from build123d import *

# Parameters (mm, degrees)
SKETCH1_W           = 18
SKETCH1_H           = 80
BOSS_EXTRUDE1_DEPTH = 5
SKETCH2_W           = 5
SKETCH2_H           = 25
BOSS_EXTRUDE2_DEPTH = 5
SKETCH3_W           = 9
SKETCH3_H           = 5
BOSS_EXTRUDE3_DEPTH = 5
SKETCH4_W           = 10
SKETCH4_H           = 5
BOSS_EXTRUDE4_DEPTH = 5
SKETCH5_R           = 2.1
CUT_EXTRUDE1_DEPTH  = 5
BOSS_EXTRUDE5_DEPTH = 5
SKETCH7_W           = 5
SKETCH7_H           = 4.2
CUT_EXTRUDE2_DEPTH  = 5


with BuildPart() as part:
    # Sketch1 → Boss-Extrude1 (new body)
    with BuildSketch(Plane.XY):
        with Locations((-9, 40)):
            Rectangle(SKETCH1_W, SKETCH1_H)
    extrude(amount=BOSS_EXTRUDE1_DEPTH)

    # Sketch2 → Boss-Extrude2 (add)
    with BuildSketch(Plane(origin=(0, 0, 0), x_dir=(-1, 0, 0), z_dir=(0, 0, -1))):
        with Locations((-2.5, 62.5)):
            Rectangle(SKETCH2_W, SKETCH2_H)
        with Locations((-2.5, 17.5)):
            Rectangle(SKETCH2_W, SKETCH2_H)
        with Locations((20.5, 17.5)):
            Rectangle(SKETCH2_W, SKETCH2_H)
        with Locations((20.5, 62.5)):
            Rectangle(SKETCH2_W, SKETCH2_H)
    extrude(amount=-BOSS_EXTRUDE2_DEPTH)

    # Sketch3 → Boss-Extrude3 (add)
    with BuildSketch(Plane.XZ):
        with Locations((-4.5, 2.5)):
            Rectangle(SKETCH3_W, SKETCH3_H)
    extrude(amount=BOSS_EXTRUDE3_DEPTH)

    # Sketch4 → Boss-Extrude4 (add)
    with BuildSketch(Plane(origin=(0, 0, 0), x_dir=(-1, 0, 0), z_dir=(0, 0, -1))):
        with Locations((5, 82.5)):
            Rectangle(SKETCH4_W, SKETCH4_H)
    extrude(amount=-BOSS_EXTRUDE4_DEPTH)

    # Sketch5 → Cut-Extrude1 (cut)
    with BuildSketch(Plane(origin=(0, 0, 0), x_dir=(-1, 0, 0), z_dir=(0, 0, -1))):
        with Locations((-2.5, 62.5)):
            Circle(SKETCH5_R)
        with Locations((-2.5, 17.5)):
            Circle(SKETCH5_R)
    extrude(amount=-CUT_EXTRUDE1_DEPTH, mode=Mode.SUBTRACT)

    # Sketch6 → Boss-Extrude5 (add)
    with BuildSketch(Plane(origin=(0, 0, 0), x_dir=(-1, 0, 0), z_dir=(0, 0, -1))):
        with BuildLine():
            Line((-5, 66.830127019), (-5, 58.169872981))
            ThreePointArc((-5, 58.169872981), (-7.5, 62.5), (-5, 66.830127019))
        make_face()
        with BuildLine():
            Line((-5, 13.169872981), (-5, 21.830127019))
            ThreePointArc((-5, 21.830127019), (-7.5, 17.5), (-5, 13.169872981))
        make_face()
    extrude(amount=-BOSS_EXTRUDE5_DEPTH)

    # Sketch7 → Cut-Extrude2 (cut)
    with BuildSketch(Plane.XY.offset(5)):
        Polygon((-13, 45), (-13, 42.1), (-13, 37.9), (-13, 35), (-3, 35), (-3, 45), align=None)
        with Locations((-15.5, 40)):
            Rectangle(SKETCH7_W, SKETCH7_H)
    extrude(amount=-CUT_EXTRUDE2_DEPTH, mode=Mode.SUBTRACT)


solid = part.part
The listing builds one solid part. Answer for the finished solid, in the listing's coordinates (mm). A direction names the side the tool comes from. Coordinates: 2 decimals unless noted, no trailing zeros. Order: outer loops, then holes, each group sorted by start corner. A loop starts at its lowest first (then second) coordinate and runs counter-clockwise, first axis right, second up. Notation, with made-up numbers: M 47.5,-22.5 L 70.5,-22.5 A28 ccw 70.5,9.5 Z; hole C -2.5,61.5 d1. An arc over 180 degrees is marked long. Use CSV: the item, a comma, the result in double quotes.
Q1. Determine the mould class of faces 5 (the flat face through (-20, 30, 2)), 6 (the flat face through (-23, 62, 2)), 7 (the cylindrical face through (1.37, 19.27, 2.46)) for opening direction X: pulls with the +X half, pulls with the -X half, needs draft (parallel to the pull), parting line crosses it, or undercut.
Here are the results:
face 5,"needs draft"
face 6,"pulls with the -X half"
face 7,"undercut"
Q2. Section C-C (y = 62.5) is taken. Determine the outline of the cut face in (x, z), then the cut area to 4 significant figures.
Here are the results:
outline,"M -23,0 L 0.4,0 L 0.4,5 L -23,5 Z; M 4.6,0 L 7.5,0 L 7.5,5 L 4.6,5 Z"
area,"131.5 mm2"
Q3. Section B-B (x = 2.5) is taken. Determine the outline of the cut face in (y, z).
Here are the results:
outline,"M 5,0 L 15.4,0 L 15.4,5 L 5,5 Z; M 19.6,0 L 30,0 L 30,5 L 19.6,5 Z; M 50,0 L 60.4,0 L 60.4,5 L 50,5 Z; M 64.6,0 L 75,0 L 75,5 L 64.6,5 Z"
Q4. Straight lines are drawn through the part: L1, parallel to Y at x = 2.5, z = 1; L2, parallel to Y at x = -19.5, z = 3.4; L3, parallel to Y at x = -11.5, z = 0.3. For each, find the intervals that lie inside material, in ascending order.
Here are the results:
L1,"5 to 15.4, 19.6 to 30, 50 to 60.4, 64.6 to 75"
L2,"5 to 30, 50 to 75"
L3,"0 to 35, 45 to 80"
Q5. A tool of negligible diameter and unlimited length cuts with its end or side. For faces 1 (the flat face through (-14, 0, 2)), 2 (the flat face through (-16, 37.9, 3)), 3 (the flat face through (-13, 36, 3)), 4 (the flat face through (0, 0, 2)), from which of +Z, -Z, +X, -X, +Y, -Y can it reach the whole face along a straight path? Write none if from no direction.
Here are the results:
face 1,"+Z, -Z, -X, -Y"
face 2,"+Z, -Z, -X"
face 3,"+Z, -Z"
face 4,"+Z, -Z, +X, -Y"
Q6. Given pin 1 Ø1.5 at (x, z) = (2.5, 2.5) entering from -Y; pin 2 Ø2.5 at (y, z) = (-1, 3) entering from +X; pin 3 Ø1.5 at (x, z) = (-19, 1) entering from +Y, each flat-ended and moving along its own axis, determine where each tip first touches the part or whether it passes through.
Here are the results:
pin 1,"y = 5"
pin 2,"x = 0"
pin 3,"y = 75"
Q7. Section D-D (z = 0.9) is taken. Give the number of separate pieces and of enclosed holes in the cut face, then the cut area to 3 significant figures.
Here are the results:
separate pieces,"1"
enclosed holes,"2"
area,"1,920 mm2"
Q8. Section A-A (x = -7.5) is taken. Determine the outline of the cut face in (y, z).
Here are the results:
outline,"M -5,0 L 35,0 L 35,5 L -5,5 Z; M 45,0 L 85,0 L 85,5 L 45,5 Z"
